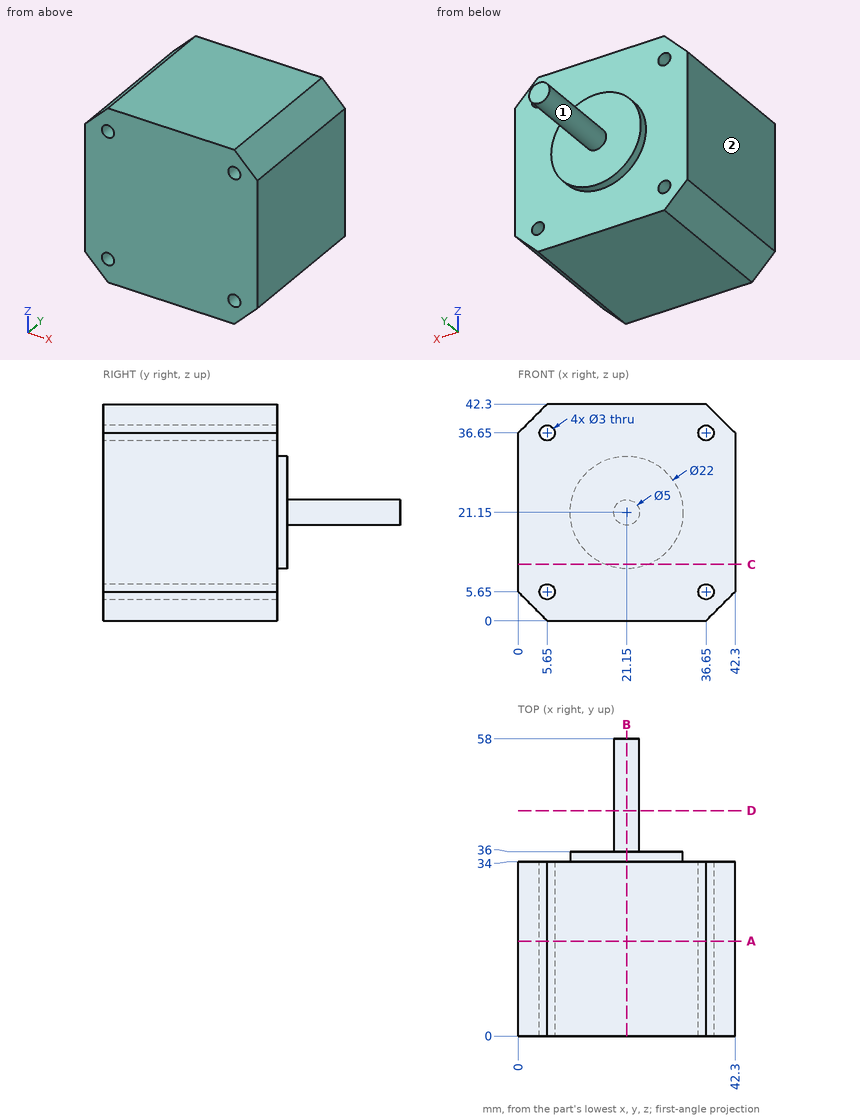
Here's the drawing with two shaded views (mm, measured from the low corner). I have some questions. A direction names the side the tool comes from. Round coordinates to 2 decimals unless told otherwise and drop trailing zeros. Loops run counter-clockwise (first coordinate to the right, second up) from the corner with the lowest first, then second, coordinate; pieces in that order, holes last.
1. Suppose I cut it at B-B, the plane x = 21.15. Please give me the cut outline in (y, z).
Answers:
outline: (0, 0) - (34, 0) - (34, 10.15) - (36, 10.15) - (36, 18.65) - (58, 18.65) - (58, 23.65) - (36, 23.65) - (36, 32.15) - (34, 32.15) - (34, 42.3) - (0, 42.3) - close
2. Will these pins go through, and if not, where does the flat tip stop? pin 1 (2.5 mm diameter, centred on x = 36.65, z = 5.65, fed in from +Y); pin 2 (5 mm diameter, centred on y = 38, z = 28, fed in from -X); pin 3 (5 mm diameter, centred on x = 5.65, z = 36.65, fed in from +Y).
Answers:
pin 1: passes through
pin 2: stops at x = 11.54
pin 3: stops at y = 34
3. If I drill on probe 1 along Z at (x, y) = (5.65, 21.5); probe 2 along Z at (x, y) = (5.5, 9.5); probe 3 along Y at (x, z) = (7, 18), over which ranges is the centre line in solid material (lowest first)?
Answers:
probe 1: z = 0 to 4.15, 7.15 to 35.15, 38.15 to 42.3
probe 2: z = 0.15 to 4.16, 7.14 to 35.16, 38.14 to 42.15
probe 3: y = 0 to 34
4. Suppose I cut it at D-D, the plane y = 44. Please give me the cut outline in (x, z), and give its area (3 significant figures).
Answers:
outline: circle Ø5 at (21.15, 21.15)
area: 19.6 mm2
5. Suppose I cut it at C-C, the plane z = 11. Please give me the cut outline in (x, y).
Answers:
outline: (0, 0) - (42.3, 0) - (42.3, 34) - (25.39, 34) - (25.39, 36) - (16.91, 36) - (16.91, 34) - (0, 34) - close
6. Suppose I cut it at A-A, the plane y = 18.5. Please give me the cut outline in (x, z), and give its area (3 significant figures).
Answers:
outline: (0, 5.65) - (5.65, 0) - (36.65, 0) - (42.3, 5.65) - (42.3, 36.65) - (36.65, 42.3) - (5.65, 42.3) - (0, 36.65) - close; hole circle Ø3 at (5.65, 5.65); hole circle Ø3 at (5.65, 36.65); hole circle Ø3 at (36.65, 5.65); hole circle Ø3 at (36.65, 36.65)
area: 1,700 mm2
7. For the marked faces 1 and 2, which set-ups out of +Z, -Z, +X, -X, +Y, -Y let a thin tool reach every point of the face, with its end or its side?
Answers:
face 1: +Y
face 2: +Z, -Z, -X, +Y, -Y
